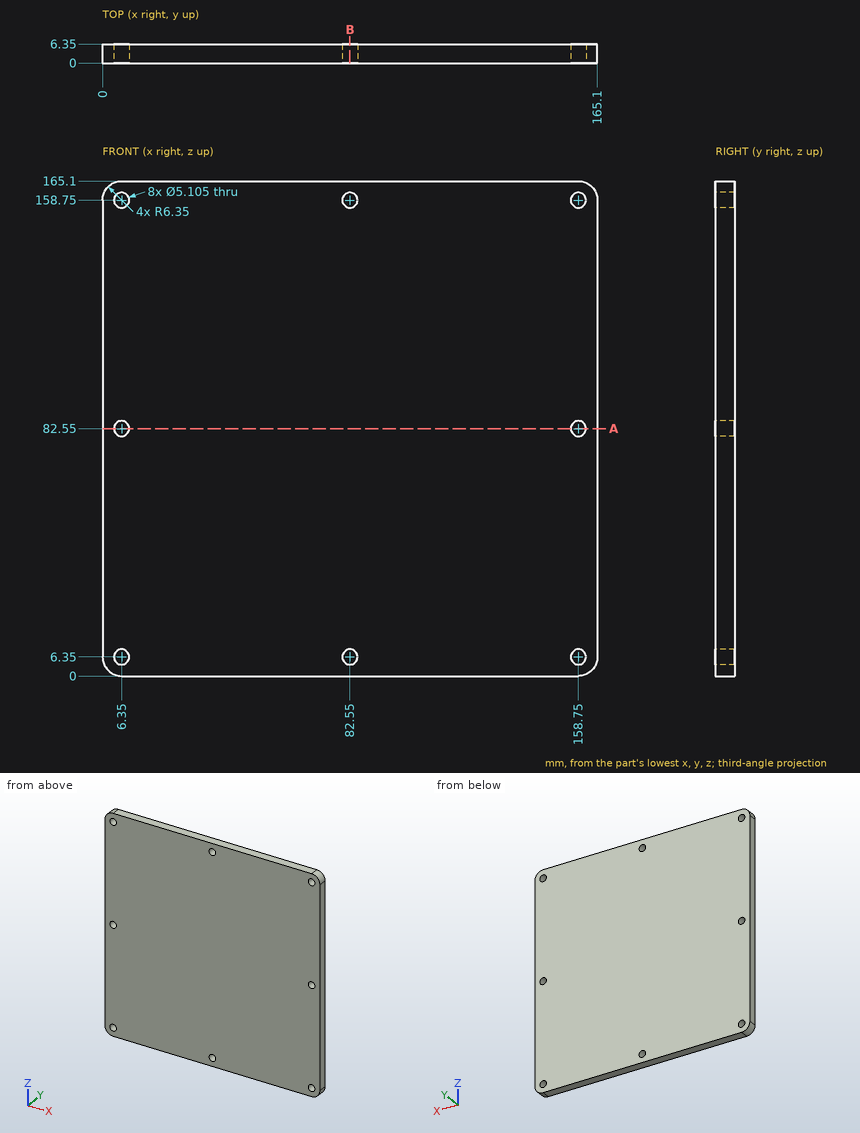
Source: three-view drawing plus pictorial views. Frame: mm from the lowest corner of the part. Coordinates: 2 decimals unless noted, no trailing zeros. Loops run counter-clockwise (first coordinate to the right, second up) from the corner with the lowest first, then second, coordinate; pieces in that order, holes last. Notation, with made-up numbers: (31.25, 87) - (38.25, 87) arc R23 cw to (38.25, 119) - close; hole circle Ø6 at (75, 12.25). An arc over 180 degrees is marked (long way). One line per item, written item: value. Start each with the question number.
1. Section A-A (z = 82.55). Return the cut outline in (x, y).
2. Section B-B (x = 82.55). Return the cut outline in (y, z).
3. Ray query, L1, parallel to Z at x = 158.5, y = 0.5; L2, parallel to X at y = 4.75, z = 6.35; L3, parallel to Z at x = 82.55, y = 2.25. Return the intervals inside material, ascending.
4. Contact query for a flat-ended pin moving along its axis: P1, Ø4.5, axis at x = 82.55, z = 6.35, coming from the -Y side. Output: stop coordinate, or through.
Verdict:
1. outline: (0, 0) - (3.8, 0) - (3.8, 6.35) - (0, 6.35) - close; (8.9, 0) - (156.2, 0) - (156.2, 6.35) - (8.9, 6.35) - close; (161.3, 0) - (165.1, 0) - (165.1, 6.35) - (161.3, 6.35) - close
2. outline: (0, 0) - (6.35, 0) - (6.35, 3.8) - (0, 3.8) - close; (0, 8.9) - (6.35, 8.9) - (6.35, 156.2) - (0, 156.2) - close; (0, 161.3) - (6.35, 161.3) - (6.35, 165.1) - (0, 165.1) - close
3. L1: z = 0 to 3.81, 8.89 to 80.01, 85.09 to 156.21, 161.29 to 165.1
3. L2: x = 0 to 3.8, 8.9 to 80, 85.1 to 156.2, 161.3 to 165.1
3. L3: z = 0 to 3.8, 8.9 to 156.2, 161.3 to 165.1
4. P1: passes through
